Check sheet for the modelled part. Datum: model origin and axes. Units: mm. A direction names the side the tool comes from. Round coordinates to 2 decimals unless told otherwise and drop trailing zeros. Order: outer loops, then holes, each group sorted by start corner. A loop starts at its lowest first (then second) coordinate and runs counter-clockwise, first axis right, second up.
(1) Sectioned sample at B-B, the plane x = 14. Enter the section's corners in (y, z), and give its area (3 significant figures).
(2) Thickness scan on probe 1 along X at (y, z) = (1.5, 13); probe 2 along X at (y, z) = (-18.5, 25); probe 3 along Y at (x, z) = (-9.5, 16). Record the ranges inside material, lowest first.
(3) Sectioned sample at C-C, the plane y = 29. Enter the section's corners in (x, z), and give its area (3 significant figures).
(4) Mould release check, pull along X, two halves, no side actions. Record for faces 1 (the flat face through (21, 0, 17)), 2 (the flat face through (27.732, -15, 17)), 3 (the flat face through (-13.597, 19, 17)): released by +X, released by -X, zero draft, split by the parting line, or undercut.
(5) Sectioned sample at A-A, the plane z = 22. Enter the section's corners in (x, y).
(6) Depth check by flat-ended pin: pin 1 (4 mm diameter, centred on x = -5.5, z = 24, fed in from -Y). Enter the tip coordinate at first touch or a pass-through.
(7) Tool access check on faces 4 (the flat face through (13.075, 25, 17)), 5 (the flat face through (3, 9, 0)), 6 (the flat face through (0, -21, 17)). Record the directions out of +Z, -Z, +X, -X, +Y, -Y that give a thin tool (end or side, any length) a straight path to the whole face; none if there is none.
```python
from build123d import *

# Parameters (mm, degrees)
F0_W     = 13.075247407
F0_H     = 11.2796872854
F1_DEPTH = 35.0964441895
F2_DEPTH = 14.6482251585


with BuildPart() as f1:
    # F0 (on Top) → F1 (new body)
    with BuildSketch(Plane.XY):
        Polygon((0, -11.2796872854), (0, 0), (13.075247407, 0), (13.075247407, 35.3304594755), (-13.5974138975, 35.3304594755), (-13.5974138975, -11.2796872854), align=None)
        Polygon((27.7324952185, 0), (13.075247407, 0), (13.075247407, -11.2796872854), (0, -11.2796872854), (0, -30.0637185574), (27.7324952185, -30.0637185574), align=None)
        with Locations((6.5376237035, -5.6398436427)):
            Rectangle(F0_W, F0_H)
    extrude(amount=F1_DEPTH)

    # F2 (add): a face of the model
    f2_faces = [f1.faces().sort_by_distance(p)[0] for p in [
        (-0.2610832453, 35.3304594755, 17.5482220948),
    ]]
    extrude(f2_faces, amount=F2_DEPTH)


solid = f1.part
```
Derived:
1. outline: (-30.06, 0) - (0, 0) - (0, 35.1) - (-30.06, 35.1) - close
1. area: 1,060 mm2
2. probe 1: x = -13.6 to 13.08
2. probe 2: x = 0 to 27.73
2. probe 3: y = -11.28 to 49.98
3. outline: (-13.6, 0) - (13.08, 0) - (13.08, 35.1) - (-13.6, 35.1) - close
3. area: 936 mm2
4. face 1: zero draft
4. face 2: released by +X
4. face 3: released by -X
5. outline: (-13.6, -11.28) - (0, -11.28) - (0, -30.06) - (27.73, -30.06) - (27.73, 0) - (13.08, 0) - (13.08, 49.98) - (-13.6, 49.98) - close
6. pin 1: stops at y = -11.28
7. face 4: +Z, -Z, +X, +Y
7. face 5: -Z, +X, -X, +Y, -Y
7. face 6: +Z, -Z, -X, -Y
